from build123d import *

# Parameters (mm, degrees)
F_8_0MM_DOWEL_HOLE1_D = 8


with BuildPart() as part:
    # Sketch1 → Revolve1 (revolve)
    with BuildSketch(Plane(origin=(0, 0, 0), x_dir=(0, 0, -1), z_dir=(1, 0, 0))):
        Polygon((0, 0), (0, -5.08), (-29.5656, -5.08), (-29.5656, -3.429), (-28.8036, -3.429), (-28.8036, -1.651), (-29.5656, -1.651), (-29.5656, 0), align=None)
    revolve(axis=Axis((0, 0, 0), (0, -1, 0)))

    # Ø8.0mm Dowel Hole1 (through all)
    with Locations(Plane(origin=(0, 0, 0), x_dir=(1, 0, 0), z_dir=(0, 1, 0))):
        with Locations((0, 0)):
            Hole(F_8_0MM_DOWEL_HOLE1_D / 2)


solid = part.part
For this review, take the finished solid that the model builds, in its own axes (mm). A direction names the side the tool comes from. Coordinates: 2 decimals unless noted, no trailing zeros. Loops run counter-clockwise (first coordinate to the right, second up) from the corner with the lowest first, then second, coordinate; pieces in that order, holes last. Notation, with made-up numbers: (49, 8) - (107, 8) arc R4 ccw to (107, 12) - close; hole circle Ø7 at (5, 45). An arc over 180 degrees is marked (long way). Return JSON: item names as keys, results as strings.
Item 1: Take a section at A-A (z = 0). Give the boundary of the cut face in (x, y).
Determined:
{"outline": "(-29.57, -5.08) - (-4, -5.08) - (-4, 0) - (-29.57, 0) - (-29.57, -1.65) - (-28.8, -1.65) - (-28.8, -3.43) - (-29.57, -3.43) - close; (4, -5.08) - (29.57, -5.08) - (29.57, -3.43) - (28.8, -3.43) - (28.8, -1.65) - (29.57, -1.65) - (29.57, 0) - (4, 0) - close"}
Item 2: Take a section at D-D (z = 12). Give the boundary of the cut face in (x, y).
Determined:
{"outline": "(-27.02, -5.08) - (27.02, -5.08) - (27.02, -3.43) - (26.18, -3.43) - (26.18, -1.65) - (27.02, -1.65) - (27.02, 0) - (-27.02, 0) - (-27.02, -1.65) - (-26.18, -1.65) - (-26.18, -3.43) - (-27.02, -3.43) - close"}
Item 3: For faces 4 (the flat face through (6, 0, 0)), 5 (the cylindrical face through (25.554, -2.528, 13.291)), list the 3-axis set-ups (+Z, -Z, +X, -X, +Y, -Y) from which the entire face can be reached by the end or side of a thin tool; tool diameter is ignored.
Determined:
{"face 4": "+Z, -Z, +X, -X, +Y", "face 5": "none"}
Item 4: Mouldability with a two-part tool opening along Y and no side actions: class faces 1 (the flat face through (6, -5.08, 0)), 2 (the cylindrical face through (0.867, -2.576, 3.905)), 3 (the flat face through (28.3, -1.651, -6.4)) as pulls with the +Y half, pulls with the -Y half, needs draft (parallel to the pull), parting line crosses it, or undercut.
Determined:
{"face 1": "pulls with the -Y half", "face 2": "needs draft", "face 3": "undercut"}
Item 5: Take a section at C-C (x = 12). Give the boundary of the cut face in (y, z), then the cut area to 3 significant figures.
Determined:
{"outline": "(-5.08, -27.02) - (-3.43, -27.02) - (-3.43, -26.18) - (-1.65, -26.18) - (-1.65, -27.02) - (0, -27.02) - (0, 27.02) - (-1.65, 27.02) - (-1.65, 26.18) - (-3.43, 26.18) - (-3.43, 27.02) - (-5.08, 27.02) - close", "area": "272 mm2"}
Item 6: Insertion check: pin 1 (2 mm diameter, centred on y = -1.5, z = -14.5, fed in from +X); pin 2 (3 mm diameter, centred on x = -14.5, y = -2.5, fed in from -Z); pin 3 (2 mm diameter, centred on x = -13, y = -2, fed in from -Z); pin 4 (10 mm diameter, centred on x = -18.5, z = -11, fed in from +Y). Each pin has a flat end and moves straight along its axis. Give the tip position at first contact, or say it passes through.
Determined:
{"pin 1": "stops at x = 26.3", "pin 2": "stops at z = -26.42", "pin 3": "stops at z = -26.99", "pin 4": "stops at y = 0"}
Item 7: For line 1 (Z direction, x = 0, y = -1.3); line 2 (Y direction, x = 24.5, z = 16); line 3 (X direction, y = -4.6, z = -3.5), list the stretches that pass through material, from the lowest coordinate up.
Determined:
{"line 1": "z = -29.57 to -4, 4 to 29.57", "line 2": "y = -5.08 to -3.43, -1.65 to 0", "line 3": "x = -29.36 to -1.94, 1.94 to 29.36"}
Item 8: Take a section at B-B (x = 0). Give the boundary of the cut face in (y, z), then the cut area to 3 significant figures.
Determined:
{"outline": "(-5.08, -29.57) - (-3.43, -29.57) - (-3.43, -28.8) - (-1.65, -28.8) - (-1.65, -29.57) - (0, -29.57) - (0, -4) - (-5.08, -4) - close; (-5.08, 4) - (0, 4) - (0, 29.57) - (-1.65, 29.57) - (-1.65, 28.8) - (-3.43, 28.8) - (-3.43, 29.57) - (-5.08, 29.57) - close", "area": "257 mm2"}
